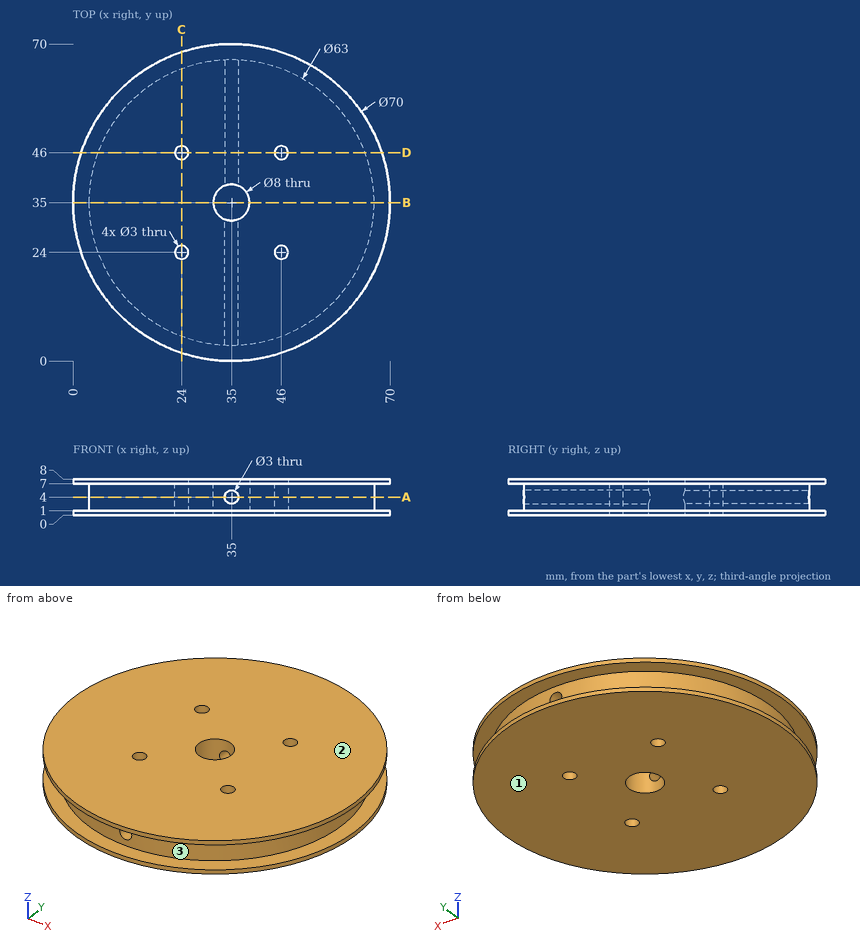
Geometry check sheet. Reference: drawing and pictorial views, mm from the part's lowest x, y, z. Give positions to 0.01 mm unless a question says otherwise; leave off trailing zeros. Order: outer loops, then holes, each group sorted by start corner. A loop starts at its lowest first (then second) coordinate and runs counter-clockwise, first axis right, second up. Notation, with made-up numbers: M -16,74.5 L 40,74.5 A18 ccw 40,86.5 Z; hole C -6.75,85 d1. An arc over 180 degrees is marked long. Answer in a Markdown table with one row per item. Add a question column.
Item 1: Gauge pin test, flat ends, axial feed: pin 1 (1.5 mm diameter, centred on x = 50.5, z = 5, fed in from +Y); pin 2 (2 mm diameter, centred on y = 31.5, z = 7, fed in from +X); pin 3 (4 mm diameter, centred on x = 50, z = 2.5, fed in from +Y). Record the tip position at first contact, or that the pin passes through.
Item 2: Section check B-B, the plane y = 35. Enter the section's corners in (x, z).
Item 3: Section check C-C, the plane x = 24. Enter the section's corners in (y, z).
Item 4: Mould release check, pull along Z, two halves, no side actions. Record for the marked faces 1, 2 and 3: released by +Z, released by -Z, zero draft, split by the parting line, or undercut.
Item 5: Section check A-A, the plane z = 4. Enter the section's corners in (x, y), and give its area (3 significant figures).
Item 6: Scan lines: probe 1 along Y at (x, z) = (46, 6); probe 2 along Z at (x, y) = (64.5, 17.5); probe 3 along Z at (x, y) = (35, 10). Record each from-to range of solid material in increasing order. Write a range as from..to.
Item 7: Section check D-D, the plane y = 46. Enter the section's corners in (x, z), and give its area (3 significant figures).
Filled sheet:
| question | item | result |
|---|---|---|
| 1 | pin 1 | stops at y = 62.83 |
| 1 | pin 2 | stops at x = 69.91 |
| 1 | pin 3 | stops at y = 67.22 |
| 2 | outline | M 0,0 L 31,0 L 31,8 L 0,8 L 0,7 L 3.5,7 L 3.5,1 L 0,1 Z; M 39,0 L 70,0 L 70,1 L 66.5,1 L 66.5,7 L 70,7 L 70,8 L 39,8 Z |
| 3 | outline | M 1.77,0 L 22.5,0 L 22.5,8 L 1.77,8 L 1.77,7 L 5.48,7 L 5.48,1 L 1.77,1 Z; M 25.5,0 L 44.5,0 L 44.5,8 L 25.5,8 Z; M 47.5,0 L 68.23,0 L 68.23,1 L 64.52,1 L 64.52,7 L 68.23,7 L 68.23,8 L 47.5,8 Z |
| 4 | face 1 | released by -Z |
| 4 | face 2 | released by +Z |
| 4 | face 3 | undercut |
| 5 | outline | M 33.5,3.54 L 33.5,31.29 A4 cw 33.5,38.71 L 33.5,66.46 A31.5 ccw Z; M 36.5,3.54 A31.5 ccw 36.5,66.46 L 36.5,38.71 A4 cw 36.5,31.29 Z; hole C 24,24 d3; hole C 24,46 d3; hole C 46,24 d3; hole C 46,46 d3 |
| 5 | area | 2,870 mm^2 |
| 6 | probe 1 | y = 5.48..22.5, 25.5..44.5, 47.5..64.52 |
| 6 | probe 2 | z = 0..1, 7..8 |
| 6 | probe 3 | z = 0..2.5, 5.5..8 |
| 7 | outline | M 1.77,0 L 22.5,0 L 22.5,8 L 1.77,8 L 1.77,7 L 5.48,7 L 5.48,1 L 1.77,1 Z; M 25.5,0 L 44.5,0 L 44.5,8 L 25.5,8 Z; M 47.5,0 L 68.23,0 L 68.23,1 L 64.52,1 L 64.52,7 L 68.23,7 L 68.23,8 L 47.5,8 Z; hole C 35,4 d3 |
| 7 | area | 432 mm^2 |
